Can you work these out from the drawing? Everything is in mm from the part's minimum corner. A direction names the side the tool comes from. Coordinates: 2 decimals unless noted, no trailing zeros. Loops run counter-clockwise (first coordinate to the right, second up) from the corner with the lowest first, then second, coordinate; pieces in that order, holes last. Notation, with made-up numbers: (65, -27.75) -> (106, -27.75) arc R11 ccw to (106, -14.75) -> close; hole circle Ø8 at (25.25, 81). An arc over 180 degrees is marked (long way). Put each result on its own line as item: value. Start each with the question number.
Item 1: Will these pins go through, and if not, where does the flat tip stop? P1, Ø4.5, axis at y = 49.25, z = 42, coming from the +X side; P2, Ø5.5, axis at y = 12.75, z = 42, coming from the -X side.
Item 2: For the marked faces 5 and 6, which set-ups out of +Z, -Z, +X, -X, +Y, -Y let a thin tool reach every point of the face, with its end or its side?
Item 3: If we section it at C-C on z = 42: Please give me the cut outline in (x, y), plus the area to 3 significant figures.
Item 4: We'd pull the mould along Y, two halves only. Please class the marked faces 1, 2, 3 and 4: pulls with the +Y half, pulls with the -Y half, needs draft (parallel to the pull), parting line crosses it, or undercut.
Item 5: If we section it at A-A on y = 31: Please give me the cut outline in (x, z), plus the area to 3 significant figures.
Item 6: If we section it at B-B on x = 44: Please give me the cut outline in (y, z).
Item 7: Please list where these lines run through material, in increasing order: L1, parallel to X at y = 31, z = 1.2; L2, parallel to Z at x = 76.35, y = 12.75; L3, parallel to Y at x = 19, z = 1.1. Write a range as from..to.
Item 8: If we section it at D-D on y = 12.75: Please give me the cut outline in (x, z), plus the area to 3 significant figures.
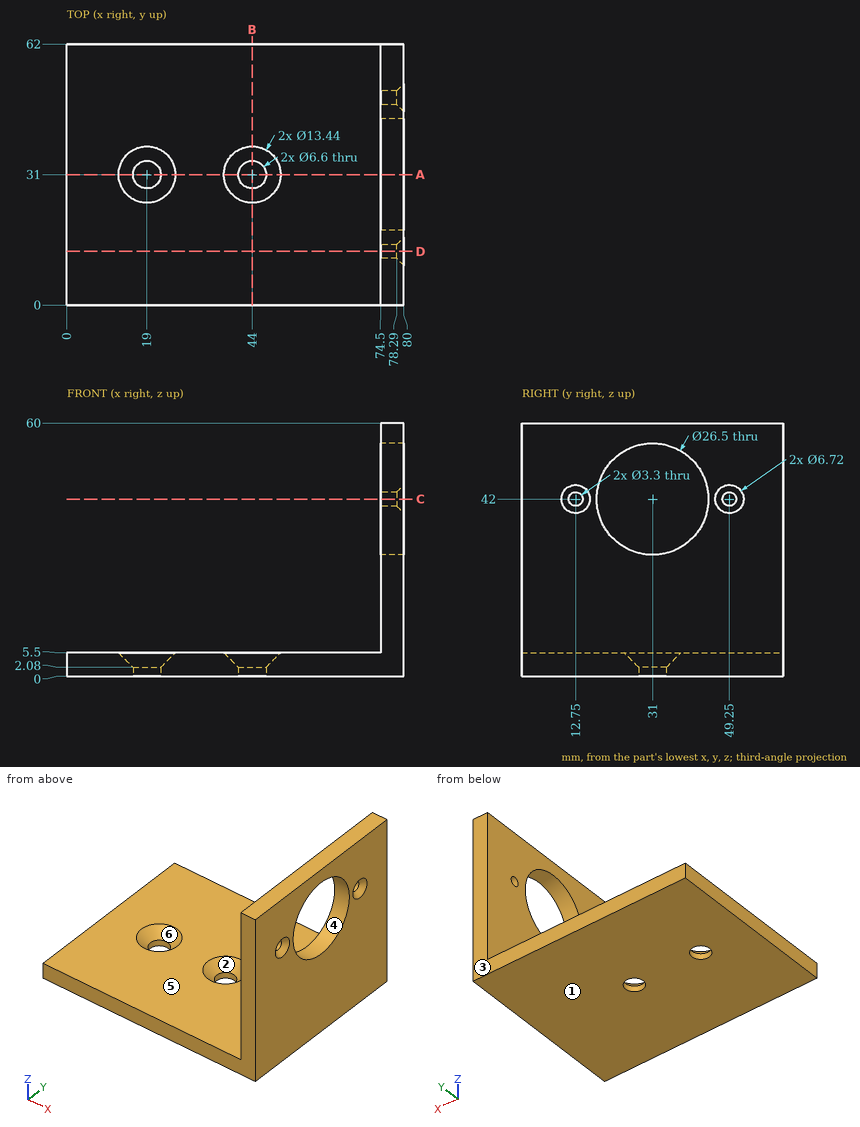
Solutions:
1. P1: x = 78.89
1. P2: x = 74.5
2. face 5: +Z, -X, +Y, -Y
2. face 6: +Z
3. outline: (74.5, 0) -> (80, 0) -> (80, 9.39) -> (78.29, 11.1) -> (74.5, 11.1) -> close; (74.5, 14.4) -> (78.29, 14.4) -> (80, 16.11) -> (80, 17.75) -> (74.5, 17.75) -> close; (74.5, 44.25) -> (80, 44.25) -> (80, 45.89) -> (78.29, 47.6) -> (74.5, 47.6) -> close; (74.5, 50.9) -> (78.29, 50.9) -> (80, 52.61) -> (80, 62) -> (74.5, 62) -> close
3. area: 153 mm^2
4. face 1: needs draft
4. face 2: undercut
4. face 3: pulls with the +Y half
4. face 4: undercut
5. outline: (0, 0) -> (15.7, 0) -> (15.7, 2.08) -> (12.28, 5.5) -> (0, 5.5) -> close; (22.3, 0) -> (40.7, 0) -> (40.7, 2.08) -> (37.28, 5.5) -> (25.72, 5.5) -> (22.3, 2.08) -> close; (47.3, 0) -> (80, 0) -> (80, 28.75) -> (74.5, 28.75) -> (74.5, 5.5) -> (50.72, 5.5) -> (47.3, 2.08) -> close; (74.5, 55.25) -> (80, 55.25) -> (80, 60) -> (74.5, 60) -> close
5. area: 498 mm^2
6. outline: (0, 0) -> (27.7, 0) -> (27.7, 2.08) -> (24.28, 5.5) -> (0, 5.5) -> close; (34.3, 0) -> (62, 0) -> (62, 5.5) -> (37.72, 5.5) -> (34.3, 2.08) -> close
7. L1: 0..15.7, 22.3..40.7, 47.3..80
7. L2: 0..40.35, 43.65..60
7. L3: 0..27.7, 34.3..62
8. outline: (0, 0) -> (80, 0) -> (80, 38.64) -> (78.29, 40.35) -> (74.5, 40.35) -> (74.5, 5.5) -> (0, 5.5) -> close; (74.5, 43.65) -> (78.29, 43.65) -> (80, 45.36) -> (80, 60) -> (74.5, 60) -> close
8. area: 719 mm^2
